from build123d import *

# Parameters (mm, degrees)
SKETCH1_R           = 20
SKETCH1_R_2         = 2.5
BOSS_EXTRUDE1_DEPTH = 1.5
SKETCH2_R           = 20
SKETCH2_R_2         = 18.5
BOSS_EXTRUDE2_DEPTH = 18.5
SKETCH4_W           = 5
SKETCH4_H           = 2
BOSS_EXTRUDE3_DEPTH = 20
CIRPATTERN2_COUNT   = 24
CHAMFER4_SIZE       = 4
CHAMFER4_SIZE2      = 6.92820323
CHAMFER5_SIZE       = 4
CHAMFER5_SIZE2      = 6.92820323


with BuildPart() as part:
    # Sketch1 → Boss-Extrude1 (new body)
    with BuildSketch(Plane.XY):
        Circle(SKETCH1_R)
        Circle(SKETCH1_R_2, mode=Mode.SUBTRACT)
    extrude(amount=BOSS_EXTRUDE1_DEPTH)

    # Sketch2 → Boss-Extrude2 (add)
    with BuildSketch(Plane.XY.offset(1.5)):
        Circle(SKETCH2_R)
        Circle(SKETCH2_R_2, mode=Mode.SUBTRACT)
    extrude(amount=BOSS_EXTRUDE2_DEPTH)

    # Sketch4 → Boss-Extrude3 (add)
    with BuildSketch(Plane(origin=(0, 0, 0), x_dir=(-1, 0, 0), z_dir=(0, 0, -1))):
        with Locations((-21.5, 0)):
            Rectangle(SKETCH4_W, SKETCH4_H)
    boss_extrude3 = extrude(amount=-BOSS_EXTRUDE3_DEPTH)

    # CirPattern2: Boss-Extrude3 ×24 about axis
    cirpattern2_axis = Axis((0, 0, 0), (0, 0, 1))
    for i in range(1, CIRPATTERN2_COUNT):
        add(boss_extrude3.rotate(cirpattern2_axis, i * 360 / CIRPATTERN2_COUNT))

    # Chamfer4
    chamfer4_edges = [part.edges().sort_by_distance(p)[0] for p in [
        (6.211657082, -23.182219831, 20),
        (0, -24, 20),
        (-6.211657082, -23.182219831, 20),
        (-12, -20.784609691, 20),
        (-16.970562748, -16.970562748, 20),
        (-20.784609691, -12, 20),
        (24, 0, 20),
        (-23.182219831, -6.211657082, 20),
        (-24, 0, 20),
        (-23.182219831, 6.211657082, 20),
        (-20.784609691, 12, 20),
        (-16.970562748, 16.970562748, 20),
        (-12, 20.784609691, 20),
        (-6.211657082, 23.182219831, 20),
        (0, 24, 20),
        (6.211657082, 23.182219831, 20),
        (12, 20.784609691, 20),
        (16.970562748, 16.970562748, 20),
        (23.182219831, -6.211657082, 20),
        (20.784609691, 12, 20),
        (23.182219831, 6.211657082, 20),
        (20.784609691, -12, 20),
        (16.970562748, -16.970562748, 20),
        (12, -20.784609691, 20),
    ]]
    chamfer4_side = [part.faces().sort_by_distance(p)[0] for p in [
        (-21.987492178, -0.32117749, 20),
    ]]
    chamfer(chamfer4_edges, length=CHAMFER4_SIZE, length2=CHAMFER4_SIZE2, reference=chamfer4_side[0])

    # Chamfer5
    chamfer5_edges = [part.edges().sort_by_distance(p)[0] for p in [
        (6.211657082, -23.182219831, 0),
        (0, -24, 0),
        (-6.211657082, -23.182219831, 0),
        (-12, -20.784609691, 0),
        (-16.970562748, -16.970562748, 0),
        (24, 0, 0),
        (-20.784609691, -12, 0),
        (-23.182219831, -6.211657082, 0),
        (-24, 0, 0),
        (-23.182219831, 6.211657082, 0),
        (-20.784609691, 12, 0),
        (-16.970562748, 16.970562748, 0),
        (-12, 20.784609691, 0),
        (-6.211657082, 23.182219831, 0),
        (0, 24, 0),
        (6.211657082, 23.182219831, 0),
        (12, 20.784609691, 0),
        (23.182219831, -6.211657082, 0),
        (16.970562748, 16.970562748, 0),
        (20.784609691, 12, 0),
        (23.182219831, 6.211657082, 0),
        (20.784609691, -12, 0),
        (16.970562748, -16.970562748, 0),
        (12, -20.784609691, 0),
    ]]
    chamfer5_side = [part.faces().sort_by_distance(p)[0] for p in [
        (-21.987492178, -0.32117749, 0),
    ]]
    chamfer(chamfer5_edges, length=CHAMFER5_SIZE, length2=CHAMFER5_SIZE2, reference=chamfer5_side[0])


solid = part.part
Geometry: final body of the model. Coordinates: model frame, mm. A direction names the side the tool comes from. Give positions to 0.01 mm unless a question says otherwise; leave off trailing zeros. Loops run counter-clockwise (first coordinate to the right, second up) from the corner with the lowest first, then second, coordinate; pieces in that order, holes last. Notation, with made-up numbers: M 75.25,49 L 92.25,49 A18 ccw 92.25,56 Z; hole C 1.5,5 d7. An arc over 180 degrees is marked long. Put each result on its own line as item: value. Start each with the question number.
1) Contact query for flat-ended pins moving along their axis: pin 1 (10 mm diameter, centred on y = -7, z = 9.5, fed in from -X); pin 2 (3 mm diameter, centred on x = -22, z = 11, fed in from +Y); pin 3 (1.2 mm diameter, centred on y = -21.5, z = 8, fed in from -X); pin 4 (8 mm diameter, centred on x = -7.5, y = -17.5, fed in from -Z). Output: stop coordinate, or through.
2) Ray query, line 1 along Y through (x, z) = (0, 12.75); line 2 along Z through (x, y) = (-8, 16); line 3 along Y through (x, z) = (-8, 17.5). Return the intervals inside material, ascending.
3) Access query for faces 1 (the cylindrical face through (12, -16, 10)), 2 (the flat face through (-22, 1, 10)), 3 (the cylindrical face through (19.83, 2.59, 9.86)), 4 (the cylindrical face through (-2.633, -19.826, 9.86)), 5 (the flat face through (-9.92, 19.18, 9.86)). Directions: +Z, -Z, +X, -X, +Y, -Y. A direction counts if a zero-diameter tool reaches every point of the face in a straight line with its end or side. Return the directions, or none.
4) Pull-direction query (X, two-part tool) for faces 6 (the flat face through (-16.98, -16.96, 9.96)), 7 (the flat face through (-4.616, -21.092, 9.86)), 8 (the flat face through (12.01, 20.78, 9.96)); classes: pulls with the +X half, pulls with the -X half, needs draft (parallel to the pull), parting line crosses it, or undercut.
5) Cut plane A-A (x = 0). Output: boundary loops of the cut face in (y, z), then the cut area to 3 significant figures.
Verdict:
1. pin 1: x = -23.44
1. pin 2: y = 12.49
1. pin 3: x = -11.8
1. pin 4: z = 0
2. line 1: -24 to -18.5, 18.5 to 24
2. line 2: 0 to 1.5
2. line 3: -18.33 to -16.68, 16.68 to 18.33
3. face 1: +Z, -Z
3. face 2: +Z, -Z, -X
3. face 3: +Z, -Z, +X
3. face 4: +Z, -Z, -Y
3. face 5: +Z, -Z, +Y
4. face 6: pulls with the -X half
4. face 7: undercut
4. face 8: pulls with the +X half
5. outline: M -24,6.93 L -20,0 L -2.5,0 L -2.5,1.5 L -18.5,1.5 L -18.5,20 L -20,20 L -24,13.07 Z; M 2.5,0 L 20,0 L 24,6.93 L 24,13.07 L 20,20 L 18.5,20 L 18.5,1.5 L 2.5,1.5 Z
5. area: 213 mm2
